Autodesk Inventor part; units mm, degrees
ref_plane "YZ Plane" through (0, 0, 0) normal (1, 0, 0) x (0, 1, 0)
ref_plane "XZ Plane" through (0, 0, 0) normal (0, 1, 0) x (-1, 0, 0)
ref_plane "XY Plane" through (0, 0, 0) normal (0, 0, 1) x (1, 0, 0)
sketch "草圖1" plane through (0, 0, 0) normal (0, 1, 0) x (-1, 0, 0)
  line L0 (0, 0) -> (9, 0)
  line L1 (9, 0) -> (9, 13.5)
  line L2 (0, 13.5) -> (0, 0)
  line L3 (2, 12) -> (2, 3)
  line L4 (2, 3) -> (7, 3)
  line L5 (7, 3) -> (7, 12)
  line L6 (9, 13.5) -> (7.1, 13.5)
  line L7 (7, 12) -> (6.85, 12)
  line L8 (7.1, 13.5) -> (6.85, 12)
  line L9 (4.5, 3) -> (4.5, 0)
  line L10 (0, 13.5) -> (1.9, 13.5)
  line L11 (2, 12) -> (2.15, 12)
  line L12 (1.9, 13.5) -> (2.15, 12)
  dimension "d0" = 13.5
  dimension "d1" = 9
  dimension "d2" = 5
  dimension "d3" = 9
  dimension "d4" = 1.5
  dimension "d5" = 2
  dimension "d6" = 1.9
  dimension "d7" = 0.15
  dimension "d8" = 2
  dimension "d9" = 5
extrude "擠出1" add sketch "草圖1" along normal blind 3
properties part number "夾持器"
CAD build for the part. Positions are in the model's coordinates, mm. A direction names the side the tool comes from. Give positions to 0.01 mm unless a question says otherwise; leave off trailing zeros. Order: outer loops, then holes, each group sorted by start corner. A loop starts at its lowest first (then second) coordinate and runs counter-clockwise, first axis right, second up. Notation, with made-up numbers: (55, 18) -> (108, 18) arc R14 ccw to (108, 40) -> close; hole circle Ø7 at (69.25, 54.25). An arc over 180 degrees is marked (long way). Return JSON: item names as keys, results as strings.
Q1. Drill centre lines: line 1 (X direction, y = 0.8, z = 8.5); line 2 (Z direction, x = -4.5, y = 2.45); line 3 (X direction, y = 1.3, z = 12.25). Where is each one in solid material? Low to high.
Working result:
{"line 1": "-9 to -7, -2 to 0", "line 2": "0 to 3", "line 3": "-9 to -6.89, -2.11 to 0"}
Q2. Saw through at C-C (x = -6). Write the cut outline in (y, z).
Working result:
{"outline": "(0, 0) -> (3, 0) -> (3, 3) -> (0, 3) -> close"}
Q3. Saw through at B-B (y = 2.15). Write the cut outline in (x, z).
Working result:
{"outline": "(-9, 0) -> (0, 0) -> (0, 13.5) -> (-1.9, 13.5) -> (-2.15, 12) -> (-2, 12) -> (-2, 3) -> (-7, 3) -> (-7, 12) -> (-6.85, 12) -> (-7.1, 13.5) -> (-9, 13.5) -> close"}
Q4. Saw through at A-A (z = 8.75). Write the cut outline in (x, y), then the cut area to 3 significant figures.
Working result:
{"outline": "(-9, 0) -> (-7, 0) -> (-7, 3) -> (-9, 3) -> close; (-2, 0) -> (0, 0) -> (0, 3) -> (-2, 3) -> close", "area": "12.0 mm²"}
Q5. Mould opens along Z. For faces 1 (the face through (-4, 1, 0)), 2 (the face through (-2, 1, 8)), 3 (the face through (-7, 1, 7)), 4 (the face through (-2.023, 1.479, 12.76)) say: pulls with the +Z half, pulls with the -Z half, needs draft (parallel to the pull), parting line crosses it, or undercut.
Working result:
{"face 1": "pulls with the -Z half", "face 2": "undercut", "face 3": "undercut", "face 4": "pulls with the +Z half"}
Q6. Which spindle directions (+Z, -Z, +X, -X, +Y, -Y) get a long thin tool onto all of the face, cutting with end or side? Do faces 5 (the face through (-9, 1, 7)), 6 (the face through (-6.977, 1.479, 12.76)). Say none if no direction does.
Working result:
{"face 5": "+Z, -Z, -X, +Y, -Y", "face 6": "+Z, +Y, -Y"}
Q7. Saw through at D-D (z = 12.75). Write the cut outline in (x, y) (3 decimals).
Working result:
{"outline": "(-9, 0) -> (-6.975, 0) -> (-6.975, 3) -> (-9, 3) -> close; (-2.025, 0) -> (0, 0) -> (0, 3) -> (-2.025, 3) -> close"}
